Work out the finished part from the listing and answer in its coordinate system (mm). A direction names the side the tool comes from. Give positions to 0.01 mm unless a question says otherwise; leave off trailing zeros. Write each loop counter-clockwise with the first axis right and the second up, starting at its lowest first coordinate (ties: lowest second). Pieces come first, ordered by that corner, then holes. Notation, with made-up numbers: (45.5, 77.25) -> (64.5, 77.25) arc R23 cw to (64.5, 86.25) -> close; hole circle Ø9 at (22.25, 40). An arc over 180 degrees is marked (long way). Write item = value, one per line. Start each with the question number.
from build123d import *

# Parameters (mm, degrees)
SKETCH1_R           = 7.5
BOSS_EXTRUDE1_DEPTH = 60
SKETCH2_R           = 1.9
CUT_EXTRUDE1_DEPTH  = 5.2
CUT_EXTRUDE2_START  = -5.2
SKETCH3_R           = 1.9
CUT_EXTRUDE2_DEPTH  = 5.2
SKETCH4_R           = 2.35
CUT_EXTRUDE3_DEPTH  = 0.8
CUT_EXTRUDE4_START  = -0.8
SKETCH5_R           = 2.35
CUT_EXTRUDE4_DEPTH  = 0.8


with BuildPart() as part:
    # Sketch1 → Boss-Extrude1 (new body)
    with BuildSketch(Plane(origin=(0, 0, 0), x_dir=(1, 0, 0), z_dir=(0, 1, 0))):
        with Locations(Location((0, 0, 0), (0, 0, 270))):
            Circle(SKETCH1_R)
    extrude(amount=BOSS_EXTRUDE1_DEPTH)

    # Sketch2 → Cut-Extrude1 (cut)
    with BuildSketch(Plane(origin=(0, 60, 0), x_dir=(1, 0, 0), z_dir=(0, 1, 0))):
        with Locations(Location((0, 0, 0), (0, 0, 270))):
            Circle(SKETCH2_R)
    extrude(amount=-CUT_EXTRUDE1_DEPTH, mode=Mode.SUBTRACT)

    # Sketch3 → Cut-Extrude2 (cut)
    with BuildSketch(Plane.XZ.offset(CUT_EXTRUDE2_START)):
        with Locations(Location((0, 0, 0), (0, 0, 90))):
            Circle(SKETCH3_R)
    extrude(amount=CUT_EXTRUDE2_DEPTH, mode=Mode.SUBTRACT)

    # Sketch4 → Cut-Extrude3 (cut)
    with BuildSketch(Plane(origin=(0, 60, 0), x_dir=(1, 0, 0), z_dir=(0, 1, 0))):
        with Locations(Location((0, 0, 0), (0, 0, 270))):
            Circle(SKETCH4_R)
    extrude(amount=-CUT_EXTRUDE3_DEPTH, mode=Mode.SUBTRACT)

    # Sketch5 → Cut-Extrude4 (cut)
    with BuildSketch(Plane.XZ.offset(CUT_EXTRUDE4_START)):
        with Locations(Location((0, 0, 0), (0, 0, 90))):
            Circle(SKETCH5_R)
    extrude(amount=CUT_EXTRUDE4_DEPTH, mode=Mode.SUBTRACT)


solid = part.part
(1) Each of these flat-tipped pins is pushed along its axis until it touches: pin 1 (3 mm diameter, centred on x = 0, z = 0, fed in from -Y); pin 2 (5 mm diameter, centred on y = 29.5, z = -6, fed in from -X); pin 3 (2 mm diameter, centred on x = 4.5, y = 31.5, fed in from -Z). Where does it stop, or does it pass through?
(2) A cutting plane is placed at C-C, the plane y = 20.5. Write down the section's boundary in (x, z).
(3) A cutting plane is placed at A-A, the plane z = 0. Write down the section's boundary in (x, y).
(4) A cutting plane is placed at B-B, the plane x = 0. Write down the section's boundary in (y, z), then the cut area to 3 significant figures.
(5) Determine the mould class of faces 1 (the cylindrical face through (0.33, 29.58, -7.493)), 2 (the cylindrical face through (0.728, 3.031, 1.755)), 3 (the flat face through (2, 0, 2)) for opening direction Z: pulls with the +Z half, pulls with the -Z half, needs draft (parallel to the pull), parting line crosses it, or undercut.
(6) A cutting plane is placed at D-D, the plane x = -6. Write down the section's boundary in (y, z), then the cut area to 3 significant figures.
(7) Find the intervals of material crossed by line 1 along X through (y, z) = (0.4, 0); line 2 along X through (y, z) = (58.1, 0); line 3 along Y through (x, z) = (2, -1), in increasing order.
(8) For faces 4 (the cylindrical face through (-0.728, 57.031, 1.755)), 5 (the cylindrical face through (-0.71, 0.41, 2.24)), 6 (the flat face through (2, 60, 2)), determine the directions among +Z, -Z, +X, -X, +Y, -Y from which every point of the face is accessible in a straight line to the end or side of a thin tool.
Results list:
q1.pin_1 = 5.2
q1.pin_2 = -6.63
q1.pin_3 = -6.63
q2.outline = circle Ø15 at (0, 0)
q3.outline = (-7.5, 0) -> (-2.35, 0) -> (-2.35, 0.8) -> (-1.9, 0.8) -> (-1.9, 5.2) -> (1.9, 5.2) -> (1.9, 0.8) -> (2.35, 0.8) -> (2.35, 0) -> (7.5, 0) -> (7.5, 60) -> (2.35, 60) -> (2.35, 59.2) -> (1.9, 59.2) -> (1.9, 54.8) -> (-1.9, 54.8) -> (-1.9, 59.2) -> (-2.35, 59.2) -> (-2.35, 60) -> (-7.5, 60) -> close
q4.outline = (0, -7.5) -> (60, -7.5) -> (60, -2.35) -> (59.2, -2.35) -> (59.2, -1.9) -> (54.8, -1.9) -> (54.8, 1.9) -> (59.2, 1.9) -> (59.2, 2.35) -> (60, 2.35) -> (60, 7.5) -> (0, 7.5) -> (0, 2.35) -> (0.8, 2.35) -> (0.8, 1.9) -> (5.2, 1.9) -> (5.2, -1.9) -> (0.8, -1.9) -> (0.8, -2.35) -> (0, -2.35) -> close
q4.area = 859 mm²
q5.face_1 = parting line crosses it
q5.face_2 = undercut
q5.face_3 = needs draft
q6.outline = (0, -4.5) -> (60, -4.5) -> (60, 4.5) -> (0, 4.5) -> close
q6.area = 540 mm²
q7.line_1 = -7.5 to -2.35, 2.35 to 7.5
q7.line_2 = -7.5 to -1.9, 1.9 to 7.5
q7.line_3 = 0.8 to 59.2
q8.face_4 = +Y
q8.face_5 = -Y
q8.face_6 = +Z, -Z, +X, -X, +Y
